from build123d import *

# Parameters (mm, degrees)
F0_R     = 35
F0_R_2   = 1.5
F1_DEPTH = 5
F2_R     = 2.49999
F3_D     = 3


# Not quite as in the source:
# - a fillet or chamfer is up to 0.001 mm smaller than in the source, because OpenCascade refuses the exact size


with BuildPart() as f1:
    # F0 (on Top) → F1 (new body)
    with BuildSketch(Plane.XY):
        Circle(F0_R)
        with Locations((0, -30)):
            Circle(F0_R_2, mode=Mode.SUBTRACT)
        with Locations((-30, 0)):
            Circle(F0_R_2, mode=Mode.SUBTRACT)
        with Locations((30, 0)):
            Circle(F0_R_2, mode=Mode.SUBTRACT)
        with Locations((0, 30)):
            Circle(F0_R_2, mode=Mode.SUBTRACT)
    extrude(amount=F1_DEPTH)

    # F2 (radius 2.5 in the source; OpenCascade refuses exactly that, so slightly less here)
    f2_edges = [f1.edges().sort_by_distance(p)[0] for p in [
        (-35, 0, 5),
        (-35, 0, 0),
    ]]
    fillet(f2_edges, radius=F2_R)

    # F3 (through all)
    with Locations(Plane(origin=(0, 0, 0), x_dir=(1, 0, 0), z_dir=(0, 0, -1))):
        with Locations((0, 0)):
            Hole(F3_D / 2)


solid = f1.part
Source: CAD feature listing. Evaluate the final solid. Frame: model axes, mm. Give positions to 0.01 mm unless a question says otherwise; leave off trailing zeros. Write each loop counter-clockwise with the first axis right and the second up, starting at its lowest first coordinate (ties: lowest second). Pieces come first, ordered by that corner, then holes. Notation, with made-up numbers: (47, -36) - (92, -36) arc R37 ccw to (92, 2) - close; hole circle Ø8 at (67, 82.25). An arc over 180 degrees is marked (long way). Write item = value, one per line. Start each with the question number.
Q1. Cut plane B-B, the plane z = 1.5. Return loops of the section in (x, y).
Q2. Pin query (flat end, axial travel): pin 1 Ø2.5 at (x, y) = (0, 30) entering from -Z; pin 2 Ø8 at (x, y) = (26.5, 25.5) entering from -Z; pin 3 Ø1.5 at (x, z) = (5, 2.5) entering from +Y. Return the tip coordinate at first contact, or that it passes through.
Q3. Draft query along Y for faces 1 (the cylindrical face through (1.5, -0.07, 2.53)), 2 (the flat face through (0, -7, 5)). Return one class per face: +Y half, -Y half, draft (parallel to the pull), parting line (faces both ways), or undercut.
Q4. Material intervals for probe 1 along Y at (x, z) = (0, 1.1); probe 2 along Y at (x, z) = (0, 1.7); probe 3 along Y at (x, z) = (-30, 2.25), sorted ascending.
Q5. Cut plane A-A, the plane y = 0. Give the number of separate pieces and of enclosed holes in the cut face, then the cut area to 3 significant figures.
Computed values:
q1.outline = circle Ø69.58 at (0, 0); hole circle Ø3 at (-30, 0); hole circle Ø3 at (0, -30); hole circle Ø3 at (0, 0); hole circle Ø3 at (0, 30); hole circle Ø3 at (30, 0)
q2.pin_1 = through
q2.pin_2 = 0.02
q2.pin_3 = 34.74
q3.face_1 = undercut
q3.face_2 = draft
q4.probe_1 = -34.57 to -31.5, -28.5 to -1.5, 1.5 to 28.5, 31.5 to 34.57
q4.probe_2 = -34.87 to -31.5, -28.5 to -1.5, 1.5 to 28.5, 31.5 to 34.87
q4.probe_3 = -18 to -1.5, 1.5 to 18
q5.separate_pieces = 4
q5.enclosed_holes = 0
q5.area = 300 mm²
